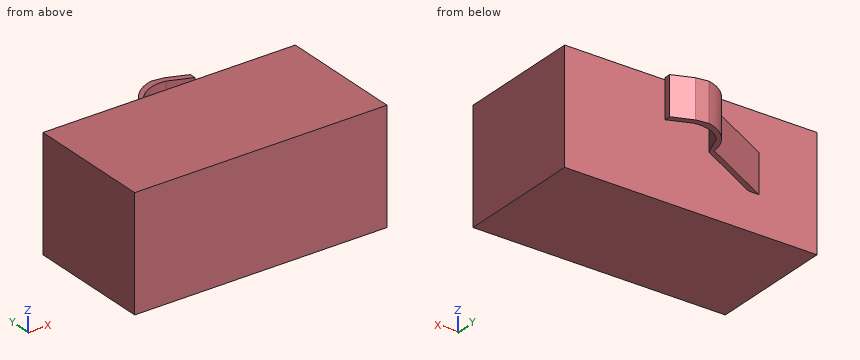
Autodesk Inventor part; units mm, degrees
ref_plane "YZ Plane" through (0, 0, 0) normal (1, 0, 0) x (0, 1, 0)
ref_plane "XZ Plane" through (0, 0, 0) normal (0, 1, 0) x (-1, 0, 0)
ref_plane "XY Plane" through (0, 0, 0) normal (0, 0, 1) x (1, 0, 0)
sketch "Sketch1" plane through (0, 0, 0) normal (0, 1, 0) x (-1, 0, 0)
  line L0 (13, -10) -> (0, -10)
  line L1 (0, -10) -> (13, -10)
  line L2 (13, -10) -> (13, -4.2)
  line L3 (13, -4.2) -> (0, -4.2)
  line L4 (0, -4.2) -> (0, -10)
  dimension "d0" = 13
  dimension "d4" = 5.8
extrude "Extrusion1" add sketch "Sketch1" along normal blind 6.5
sketch "Sketch2" plane through (0, 6.5, 0) normal (0, 1, 0) x (1, 0, 0)
  line L0 (0, 4.2) -> (0, 10)
  line L1 (0, 0) -> (0, 4.2)
  line L2 (0, 4.2) -> (0, 10)
  line L3 (0, 4.2) -> (0, 10)
  line L4 (0, 7.1) -> (-3, 7.1)
  line L5 (-3, 7.1) -> (-3, 8.1)
  line L6 (-3, 8.1) -> (-3, 6.1)
  line L7 (-3, 8.1) -> (-10, 8.1)
  line L8 (-10, 8.1) -> (-10, 6.1)
  line L9 (-10, 6.1) -> (-3, 6.1)
  line L10 (-3, 6.1) -> (-3, 8.1)
  dimension "d5" = 3
  dimension "d6" = 1
  dimension "d7" = 2
  dimension "d8" = 7
extrude "Extrusion2" add sketch "Sketch2" along normal blind 6
sketch "Sketch3" plane through (-10, 6.5, -6.1) normal (0, 0, 1) x (1, 0, 0)
  line L0 (7, 0) -> (0, 0)
  line L1 (0, 0) -> (3.7445, 1.9981)
  line L2 (3.7445, 1.9981) -> (3.8617, 1.7785)
  line L3 (3.8617, 1.7785) -> (0.5288, 0)
  arc A0 (5.3386, 3.8121) -> (3.7445, 1.9981) centre (5.7324, 1.8586) ccw
  arc A1 (5.8481, 3.4507) -> (4.2692, 2.8715) centre (5.5714, 1.7635) ccw
  line L4 (5.9577, 3.7284) -> (7.4262, 3.1492)
  line L5 (7.4262, 3.1492) -> (7.3166, 2.8715)
  line L6 (7.3166, 2.8715) -> (5.8481, 3.4507)
  line L7 (5.3386, 3.8121) -> (5.9577, 3.7284)
  line L8 (3.8617, 1.7785) -> (4.2692, 2.8715)
  line L9 (0.5288, 0) -> (0, 0)
  line L10 (7, 6) -> (0, 6)
  line L11 (0, 6) -> (7, 6)
  line L12 (7, 6) -> (7, 0)
  line L13 (7, 0) -> (0, 0)
  line L14 (0, 0) -> (0, 6)
  point P0 (10, -6.5)
  point P1 (7, 2.9964)
  point P2 (7, 3.3173)
extrude "Extrusion3" cut sketch "Sketch3" against normal blind 6 contours L0 L3 L8 A1 L6 L12 | L14 L10 L12 L4 L7 A0 L1
properties part number "WK330"
Work out the finished part from the listing and answer in its coordinate system (mm). Round coordinates to 2 decimals unless told otherwise and drop trailing zeros. Write each loop counter-clockwise with the first axis right and the second up, starting at its lowest first coordinate (ties: lowest second). Pieces come first, ordered by that corner, then holes. Notation, with made-up numbers: M 89.25,31 L 144.25,31 A13 cw 144.25,48 Z; hole C 88.25,24.5 d5. An arc over 180 degrees is marked long. Use a Markdown table: item, result.
1) Flat-ended cylindrical pins translate along their axes: pin 1 (3 mm diameter, centred on x = -8, z = -6, fed in from +Y); pin 2 (1.9 mm diameter, centred on x = -6, y = 8.5, fed in from -Z); pin 3 (1.1 mm diameter, centred on x = -7, y = 8.5, fed in from +Z). Find the tip coordinate at first contact, or state that the pin passes through.
Taken from the geometry:
| item | result |
|---|---|
| pin 1 | stops at y = 8.37 |
| pin 2 | stops at z = -8.1 |
| pin 3 | stops at z = -6.1 |
2) Consider line 1 (Y direction, x = -9.5, z = -8.45); line 2 (Y direction, x = -3.25, z = -8); line 3 (X direction, y = 9.25, z = -7.7). Determine where each line is inside the solid, lowest interval first. Write a range as [from, to].
Taken from the geometry:
| item | result |
|---|---|
| line 1 | y = [0, 6.5] |
| line 2 | y = [0, 6.5], [9.59, 9.92] |
| line 3 | x = [-6.05, -5.78] |
3) The part is cut by section B-B on z = -7.3. Give the vertices of the cut face in (x, y), plus the area to 3 significant figures.
Taken from the geometry:
| item | result |
|---|---|
| outline | M -13,0 L 0,0 L 0,6.5 L -9.47,6.5 L -6.14,8.28 L -5.73,9.37 A1.71 cw -4.15,9.95 L -3,9.5 L -3,9.82 L -4.04,10.23 L -4.66,10.31 A1.99 ccw -6.26,8.5 L -10,6.5 L -13,6.5 Z |
| area | 86.7 mm2 |
4) The part is cut by section A-A on x = -3.5. Give the vertices of the cut face in (y, z).
Taken from the geometry:
| item | result |
|---|---|
| outline | M 0,-10 L 6.5,-10 L 6.5,-4.2 L 0,-4.2 Z; M 9.69,-8.1 L 10.01,-8.1 L 10.01,-6.1 L 9.69,-6.1 Z |
5) The part is cut by section C-C on z = -9. Give the vertices of the cut face in (x, y), plus the area to 3 significant figures.
Taken from the geometry:
| item | result |
|---|---|
| outline | M -13,0 L 0,0 L 0,6.5 L -13,6.5 Z |
| area | 84.5 mm2 |
